from build123d import *

# Parameters (mm, degrees)
BOSS_EXTRUDE1_DEPTH     = 12.2
SKETCH3_R               = 0.85
CUT_EXTRUDE1_DEPTH      = 8.75
CUT_EXTRUDE2_REACH      = 14.2
SKETCH4_R               = 1.55
SKETCH5_R               = 1.55
CUT_EXTRUDE3_DEPTH      = 1
CUT_EXTRUDE3_DEPTH_BACK = 7


with BuildPart() as part:
    # Sketch2 → Boss-Extrude1 (new body)
    with BuildSketch(Plane.XY.offset(-44.970352008)):
        Polygon((-11.212990891, 70.521798878), (-11.212990891, 58.321361968), (-2.212990891, 58.321361968), (-2.212990891, 65.521798878), (3.096001096, 70.521798878), (3.096001096, 75.396798878), (-5.653998904, 75.396798878), (-5.653998904, 70.521798878), align=None)
    extrude(amount=-BOSS_EXTRUDE1_DEPTH)

    # Sketch3 → Cut-Extrude1 (cut)
    with BuildSketch(Plane.ZY.offset(5.653998904)):
        with Locations((-51.282859951, 72.195892432)):
            Circle(SKETCH3_R)
    extrude(amount=-CUT_EXTRUDE1_DEPTH, mode=Mode.SUBTRACT)

    # Sketch4 → Cut-Extrude2 (cut, up to next)
    with BuildSketch(Plane.XY.offset(-44.970352008), mode=Mode.PRIVATE) as cut_extrude2_sk1:
        with Locations((-6.712990891, 63.321361968)):
            Circle(SKETCH4_R)
    cut_extrude2_tool1 = extrude(cut_extrude2_sk1.sketch, amount=-CUT_EXTRUDE2_REACH, mode=Mode.PRIVATE) & part.part
    add(cut_extrude2_tool1.solids().sort_by_distance((-6.712991, 63.321362, -44.970352))[0], mode=Mode.SUBTRACT)

    # Sketch5 → Cut-Extrude3 (cut, two sides)
    with BuildSketch(Plane(origin=(0, 0, -57.170352008), x_dir=(-1, 0, 0), z_dir=(0, 0, -1))) as cut_extrude3_sk:
        Polygon((11.212990891, 66.612258502), (1.05514261, 66.612258502), (2.212990891, 65.521798878), (2.212990891, 58.321361968), (11.212990891, 58.321361968), align=None)
        with Locations((6.712990891, 63.321361968)):
            Circle(SKETCH5_R, mode=Mode.SUBTRACT)
    extrude(amount=CUT_EXTRUDE3_DEPTH, mode=Mode.SUBTRACT)
    extrude(cut_extrude3_sk.sketch, amount=-CUT_EXTRUDE3_DEPTH_BACK, mode=Mode.SUBTRACT)

    # Sketch7 → Cut-Revolve1 (revolve, cut)
    with BuildSketch(Plane(origin=(0, 0, -58.682859951), x_dir=(-1, 0, 0), z_dir=(0, 0, -1))):
        Polygon((11.212990891, 66.612258502), (11.212990891, 70.521798878), (9.823409812, 70.521798878), (9.273959744, 66.612258502), align=None)
    revolve(axis=Axis((-13.092990891, 78.216716655, -58.682859951), (0, -1, 0)), mode=Mode.SUBTRACT)


solid = part.part
Here's how the part is built. I have some questions about the finished solid (model axes, mm). A direction names the side the tool comes from. Coordinates: 2 decimals unless noted, no trailing zeros. Order: outer loops, then holes, each group sorted by start corner. A loop starts at its lowest first (then second) coordinate and runs counter-clockwise, first axis right, second up. Notation, with made-up numbers: (61, -35.75) -> (77, -35.75) arc R18 ccw to (77, -4.75) -> close; hole circle Ø10 at (-37, 46.25). An arc over 180 degrees is marked (long way). Answer in a Markdown table with one row per item.
(1) Thinking about a two-plate mould opening in Y: for faces 5 (the face through (-1.34, 71.68, -51.96)), 6 (the face through (-6.1, 61.6, -50.17)), 7 (the face through (-1, 75.397, -51)), 8 (the face through (0.404, 67.987, -50.985)), which applies, +Y half, -Y half, draft (parallel to the pull), parting line (faces both ways), or undercut?
Answer key:
| item | result |
|---|---|
| face 5 | undercut |
| face 6 | draft |
| face 7 | +Y half |
| face 8 | -Y half |
(2) I want a section at B-B on x = -3.25. List the corners of the cut face in (y, z) for me.
Answer key:
| item | result |
|---|---|
| outline | (58.32, -50.17) -> (66.61, -50.17) -> (66.61, -57.17) -> (75.4, -57.17) -> (75.4, -44.97) -> (58.32, -44.97) -> close; hole circle Ø1.7 at (72.2, -51.28) |
(3) I want a section at A-A on z = -49.5. List the corners of the cut face in (x, y) for me.
Answer key:
| item | result |
|---|---|
| outline | (-11.21, 58.32) -> (-2.21, 58.32) -> (-2.21, 65.52) -> (3.1, 70.52) -> (3.1, 75.4) -> (-5.65, 75.4) -> (-5.65, 70.52) -> (-11.21, 70.52) -> close; hole circle Ø3.1 at (-6.71, 63.32) |
(4) I want a section at D-D on z = -51.75. List the corners of the cut face in (x, y) for me, then the cut area to 3 significant figures.
Answer key:
| item | result |
|---|---|
| outline | (-11.21, 66.61) -> (-1.06, 66.61) -> (3.1, 70.52) -> (3.1, 71.49) -> (-5.65, 71.49) -> (-5.65, 70.52) -> (-11.21, 70.52) -> close; (-5.65, 72.91) -> (3.1, 72.91) -> (3.1, 75.4) -> (-5.65, 75.4) -> close |
| area | 78.1 mm^2 |
(5) Please list where these lines run through material, in increasing order: probe 1 along Z at (x, y) = (-8.75, 61.75); probe 2 along Y at (x, z) = (-5.75, -51.5); probe 3 along Y at (x, z) = (-5, -56.5).
Answer key:
| item | result |
|---|---|
| probe 1 | -50.17 to -44.97 |
| probe 2 | 66.61 to 70.52 |
| probe 3 | 66.61 to 75.4 |
(6) On a 3-axis mill with a long thin cutter (end or side, diameter ignored), from which of +Z, -Z, +X, -X, +Y, -Y can I reach the whole of each face in a straight line? I mean faces 1 (the face through (-7, 58.321, -48)), 2 (the face through (-6, 66.612, -54)), 3 (the face through (-8, 70.522, -51)), 4 (the face through (-2.213, 62, -48)). Say none if no direction works.
Answer key:
| item | result |
|---|---|
| face 1 | +Z, -Z, +X, -X, -Y |
| face 2 | -Z, +X, -X, -Y |
| face 3 | +Z, -Z, -X, +Y |
| face 4 | +Z, -Z, +X, -Y |
(7) I want a section at C-C on z = -53.75. List the corners of the cut face in (x, y) for me.
Answer key:
| item | result |
|---|---|
| outline | (-11.21, 66.61) -> (-1.06, 66.61) -> (3.1, 70.52) -> (3.1, 75.4) -> (-5.65, 75.4) -> (-5.65, 70.52) -> (-11.21, 70.52) -> close |
(8) Will these pins go through, and if not, where does the flat tip stop? pin 1 Ø3 at (y, z) = (68, -50) entering from +X; pin 2 Ø5.5 at (x, z) = (-7, -53) entering from -Y; pin 3 Ø2.5 at (y, z) = (73, -53.5) entering from -X.
Answer key:
| item | result |
|---|---|
| pin 1 | x = 2.01 |
| pin 2 | y = 66.61 |
| pin 3 | x = -5.65 |
